Job drawing, mm, ordinate dimensions from the low corner. One solid piece. A direction names the side the tool comes from. Coordinates: 2 decimals unless noted, no trailing zeros. Order: outer loops, then holes, each group sorted by start corner. A loop starts at its lowest first (then second) coordinate and runs counter-clockwise, first axis right, second up. Notation, with made-up numbers: M 79.25,87.5 L 96.25,87.5 A21 ccw 96.25,110.5 Z; hole C 6.5,16 d1. An arc over 180 degrees is marked long. Write item = value, one per line.
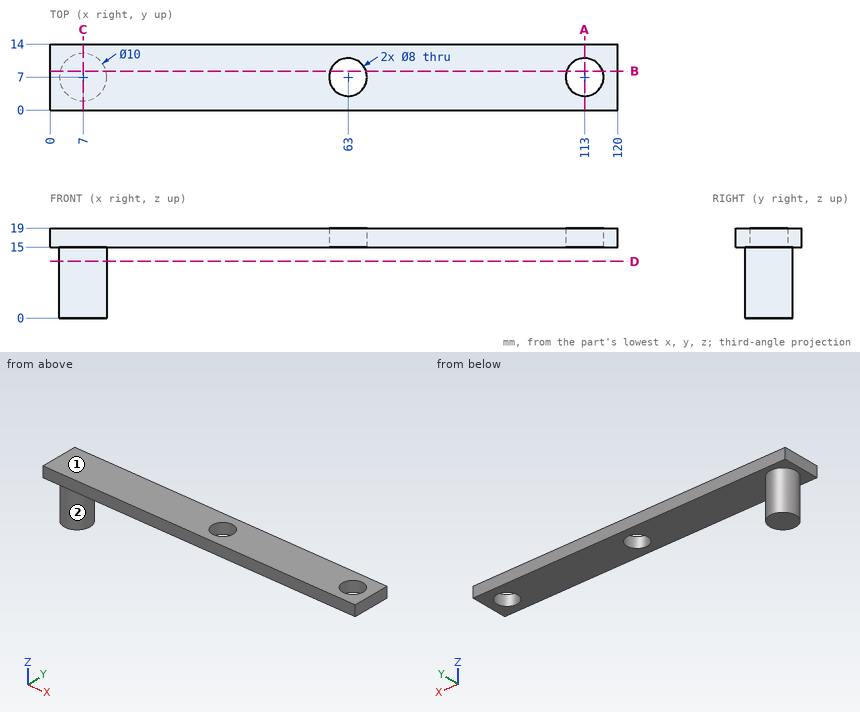
(1) Slice it at A-A, the plane x = 113. Write the cut outline in (y, z).
Evaluation:
outline = M 0,15 L 3,15 L 3,19 L 0,19 Z; M 11,15 L 14,15 L 14,19 L 11,19 Z
(2) Slice it at D-D, the plane z = 12. Write the cut outline in (x, y).
Evaluation:
outline = C 7,7 d10
(3) Wall check: line 1 (Y direction, x = 63, z = 17.6); line 2 (Z direction, x = 104, y = 5); line 3 (X direction, y = 10.5, z = 7.5). Give the ranges that are in metal, low to high. Write a range as from..to.
Evaluation:
line_1 = 0..3, 11..14
line_2 = 15..19
line_3 = 3.43..10.57
(4) Slice it at C-C, the plane x = 7. Write the cut outline in (y, z).
Evaluation:
outline = M 0,15 L 2,15 L 2,0 L 12,0 L 12,15 L 14,15 L 14,19 L 0,19 Z
(5) Slice it at B-B, the plane y = 8.25. Write the cut outline in (x, z), then the cut area to 3 significant figures.
Evaluation:
outline = M 0,15 L 2.16,15 L 2.16,0 L 11.84,0 L 11.84,15 L 59.2,15 L 59.2,19 L 0,19 Z; M 66.8,15 L 109.2,15 L 109.2,19 L 66.8,19 Z; M 116.8,15 L 120,15 L 120,19 L 116.8,19 Z
area = 564 mm²
(6) Tool access for the marked faces 1 and 2: list every direction of +Z, -Z, +X, -X, +Y, -Y with a clear straight run to the whole face (end or side of a thin tool).
Evaluation:
face_1 = +Z, +X, -X, +Y, -Y
face_2 = -Z
(7) Pin check, flat tips, straight feed: pin 1 Ø5 at (y, z) = (7, 15.5) entering from -X; pin 2 Ø10 at (x, z) = (18, 7.5) entering from +Y; pin 3 Ø6 at (y, z) = (4, 3.5) entering from +X; pin 4 Ø4 at (x, y) = (88.5, 9.5) entering from -Z. Stop position of each tip, or through.
Evaluation:
pin_1 = 0
pin_2 = through
pin_3 = 12
pin_4 = 15
